from build123d import *

# Parameters (mm, degrees)
SKETCH1_W           = 609.6
SKETCH1_H           = 228.6
BOSS_EXTRUDE1_DEPTH = 6.35
SKETCH2_R           = 2.032
CUT_EXTRUDE4_DEPTH  = 7.35
SKETCH3_R           = 4.953
CUT_EXTRUDE6_DEPTH  = 1.27
SKETCH4_R           = 2.032
CUT_EXTRUDE7_DEPTH  = 7.35
SKETCH5_R           = 4.953
CUT_EXTRUDE8_DEPTH  = 1.27


with BuildPart() as part:
    # Sketch1 → Boss-Extrude1 (new body)
    with BuildSketch(Plane.XY):
        with Locations((304.8, 114.3)):
            Rectangle(SKETCH1_W, SKETCH1_H)
    extrude(amount=BOSS_EXTRUDE1_DEPTH)

    # Sketch2 → Cut-Extrude4 (cut, through all)
    with BuildSketch(Plane.XY.offset(6.35)):
        with Locations((12.7, 203.2)):
            Circle(SKETCH2_R)
        with Locations((12.7, 107.95)):
            Circle(SKETCH2_R)
        with Locations((12.7, 12.7)):
            Circle(SKETCH2_R)
        with Locations((596.9, 12.7)):
            Circle(SKETCH2_R)
        with Locations((596.9, 107.95)):
            Circle(SKETCH2_R)
        with Locations((596.9, 203.2)):
            Circle(SKETCH2_R)
    extrude(amount=-CUT_EXTRUDE4_DEPTH, mode=Mode.SUBTRACT)

    # Sketch3 → Cut-Extrude6 (cut)
    with BuildSketch(Plane.XY.offset(6.35)):
        with Locations((12.7, 203.2)):
            Circle(SKETCH3_R)
        with Locations((12.7, 107.95)):
            Circle(SKETCH3_R)
        with Locations((12.7, 12.7)):
            Circle(SKETCH3_R)
        with Locations((596.9, 12.7)):
            Circle(SKETCH3_R)
        with Locations((596.9, 107.95)):
            Circle(SKETCH3_R)
        with Locations((596.9, 203.2)):
            Circle(SKETCH3_R)
    extrude(amount=-CUT_EXTRUDE6_DEPTH, mode=Mode.SUBTRACT)

    # Sketch4 → Cut-Extrude7 (cut, through all)
    with BuildSketch(Plane.XY.offset(6.35)):
        with Locations((34.925, 215.9)):
            Circle(SKETCH4_R)
        with Locations((142.875, 215.9)):
            Circle(SKETCH4_R)
        with Locations((250.825, 215.9)):
            Circle(SKETCH4_R)
        with Locations((358.775, 215.9)):
            Circle(SKETCH4_R)
        with Locations((466.725, 215.9)):
            Circle(SKETCH4_R)
        with Locations((574.675, 215.9)):
            Circle(SKETCH4_R)
    extrude(amount=-CUT_EXTRUDE7_DEPTH, mode=Mode.SUBTRACT)

    # Sketch5 → Cut-Extrude8 (cut)
    with BuildSketch(Plane.XY.offset(6.35)):
        with Locations((34.925, 215.9)):
            Circle(SKETCH5_R)
        with Locations((142.875, 215.9)):
            Circle(SKETCH5_R)
        with Locations((250.825, 215.9)):
            Circle(SKETCH5_R)
        with Locations((358.775, 215.9)):
            Circle(SKETCH5_R)
        with Locations((466.725, 215.9)):
            Circle(SKETCH5_R)
        with Locations((574.675, 215.9)):
            Circle(SKETCH5_R)
    extrude(amount=-CUT_EXTRUDE8_DEPTH, mode=Mode.SUBTRACT)


solid = part.part
Design review of the part built by this model. Coordinates are the model's own, in mm. Give positions to 0.01 mm unless a question says otherwise; leave off trailing zeros. Write item = value, one per line.
Q1. Draft analysis for pull direction X (two halves, no side actions). For faces 1 (the flat face through (301, 116, 0)), 2 (the cylindrical face through (469, 211.5, 5.7)), 3 (the flat face through (13, 201, 5.08)), state which applies: +X half, -X half, draft (parallel to the pull), parting line (faces both ways), or undercut.
Output values:
face_1 = draft
face_2 = undercut
face_3 = undercut
Q2. Insertion check: pin 1 (8 mm diameter, centred on x = 466.725, y = 215.9, fed in from +Z). The pin has a flat end and moves straight along its axis. Give the tip position at first contact, or say it passes through.
Output values:
pin_1 = 5.08
Q3. To check wall thickness, follow line 1 (X direction, y = 203.2, z = 3); line 2 (Y direction, x = 12.7, z = 5.65); line 3 (Y direction, x = 596.9, z = 1.15). State the ranges of each line that lie inside material, in increasing order. Write a range as [from, to].
Output values:
line_1 = [0, 10.67], [14.73, 594.87], [598.93, 609.6]
line_2 = [0, 7.75], [17.65, 103], [112.9, 198.25], [208.15, 228.6]
line_3 = [0, 10.67], [14.73, 105.92], [109.98, 201.17], [205.23, 228.6]
